```python
from build123d import *

# Parameters (mm, degrees)
SKETCH_1_W          = 103
SKETCH_1_H          = 3.03
SKETCH_2_R          = 1.5
CUT_EXTRUDE_1_DEPTH = 14.03


with BuildPart() as part:
    # Эскиз1 → Повернуть1 (revolve)
    with BuildSketch(Plane.XY):
        Polygon((0, 0), (0, 10), (103, 10), (107, 5), (119, 5), (119, 0), align=None)
        with Locations((51.5, 11.515)):
            Rectangle(SKETCH_1_W, SKETCH_1_H)
        Polygon((119, 5), (119, 0), (121, 0), (121, 110), (119, 110), align=None)
    revolve(axis=Axis((0, 0, 0), (0, 1, 0)))

    # Эскиз2 → Вырез-Вытянуть1 (cut, through all)
    with BuildSketch(Plane(origin=(0, 13.03, 0), x_dir=(1, 0, 0), z_dir=(0, 1, 0))):
        with Locations((-58, 58)):
            Circle(SKETCH_2_R)
        with Locations((58, 58)):
            Circle(SKETCH_2_R)
        with Locations((58, -58)):
            Circle(SKETCH_2_R)
        with Locations((-58, -58)):
            Circle(SKETCH_2_R)
    extrude(amount=-CUT_EXTRUDE_1_DEPTH, mode=Mode.SUBTRACT)


solid = part.part
```
Could you check a few things on this model? Use its own coordinates, in mm. A direction names the side the tool comes from. Give positions to 0.01 mm unless a question says otherwise; leave off trailing zeros. Write each loop counter-clockwise with the first axis right and the second up, starting at its lowest first coordinate (ties: lowest second). Pieces come first, ordered by that corner, then holes. Notation, with made-up numbers: (18.5, 30) -> (63.5, 30) arc R20 ccw to (63.5, 59) -> close; hole circle Ø10 at (45, 79). An arc over 180 degrees is marked (long way). Write each question's results on one line, items separated by ' | '.
1. On a 3-axis mill with a long thin cutter (end or side, diameter ignored), from which of +Z, -Z, +X, -X, +Y, -Y can I reach the whole of each face in a straight line? I mean faces 4 (the flat face through (1, 13.03, -1)), 5 (the flat face through (2, 0, -2)). Say none if no direction works.
Check sheet entries:
face 4: +Y | face 5: +Z, -Z, +X, -X, -Y
2. If we mould it in two halves opening along X, with no side actions, what happens to faces 1 (the cylindrical face through (-26.23, 55.77, 118.123)), 2 (the flat face through (89, 110, 80)), 3 (the cylindrical face through (63.974, 56.765, -100.341))? For each: released by +X, released by -X, zero draft, split by the parting line, or undercut.
Check sheet entries:
face 1: split by the parting line | face 2: zero draft | face 3: undercut
3. I want a section at C-C, the plane z = 0. Write out the boundary of the cut face in (x, y).
Check sheet entries:
outline: (-121, 0) -> (121, 0) -> (121, 110) -> (119, 110) -> (119, 5) -> (107, 5) -> (103, 10) -> (103, 13.03) -> (-103, 13.03) -> (-103, 10) -> (-107, 5) -> (-119, 5) -> (-119, 110) -> (-121, 110) -> close
4. I need wall thicknesses on L1, parallel to X at y = 74, z = 0; L2, parallel to X at y = 8, z = -58; L3, parallel to X at y = 5.75, z = -58. Which ranges of each line are inside material? Lowest first, please.
Check sheet entries:
L1: x = -121 to -119, 119 to 121 | L2: x = -106.19 to -103.91, -87.05 to -59.5, -56.5 to 56.5, 59.5 to 87.05, 103.91 to 106.19 | L3: x = -106.19 to -103.91, -89.2 to -59.5, -56.5 to 56.5, 59.5 to 89.2, 103.91 to 106.19
5. Will these pins go through, and if not, where does the flat tip stop? pin 1 Ø5 at (x, z) = (47, -3) entering from +Y; pin 2 Ø1.8 at (x, z) = (-58, 58) entering from -Y; pin 3 Ø8 at (x, y) = (-67, 90.5) entering from -Z; pin 4 Ø6 at (x, y) = (85, 96.5) entering from +Z.
Check sheet entries:
pin 1: stops at y = 13.03 | pin 2: passes through | pin 3: stops at z = -103.31 | pin 4: stops at z = 88.98
6. I want a section at B-B, the plane y = 51.5. Write out the boundary of the cut face in (x, z).
Check sheet entries:
outline: circle Ø242 at (0, 0); hole circle Ø238 at (0, 0)
7. I want a section at A-A, the plane x = 0. Write out the boundary of the cut face in (y, z).
Check sheet entries:
outline: (0, -121) -> (110, -121) -> (110, -119) -> (5, -119) -> (5, -107) -> (10, -103) -> (13.03, -103) -> (13.03, 103) -> (10, 103) -> (5, 107) -> (5, 119) -> (110, 119) -> (110, 121) -> (0, 121) -> close
